Print and shaded views of the part. All mm, measured from the part's lowest x, y and z. Coordinates: 2 decimals unless noted, no trailing zeros. Loops run counter-clockwise (first coordinate to the right, second up) from the corner with the lowest first, then second, coordinate; pieces in that order, holes last.
1) Two-plate mould, pull along Z, no slides. Class the marked faces 1, 2, 3 and 4: +Z half, -Z half, draft (parallel to the pull), parting line (faces both ways), or undercut.
2) Saw through at B-B, the plane y = 1.5. Write the cut outline in (x, z) (1 decimal), and give its area (3 significant figures).
3) Wall check: line 1 along Z through (x, y) = (5.75, 4.25) (1 decimal); line 2 along Y through (x, z) = (11.25, 2.5) (1 decimal); line 3 along X through (y, z) = (3, 4.5). Give the ranges that are in metal, low to high.
4) Pin check, flat tips, straight feed: pin 1 Ø2.5 at (x, z) = (21, 20.5) entering from -Y (3 decimals); pin 2 Ø4 at (x, z) = (7, 3.5) entering from +Y (3 decimals). Stop position of each tip, or through.
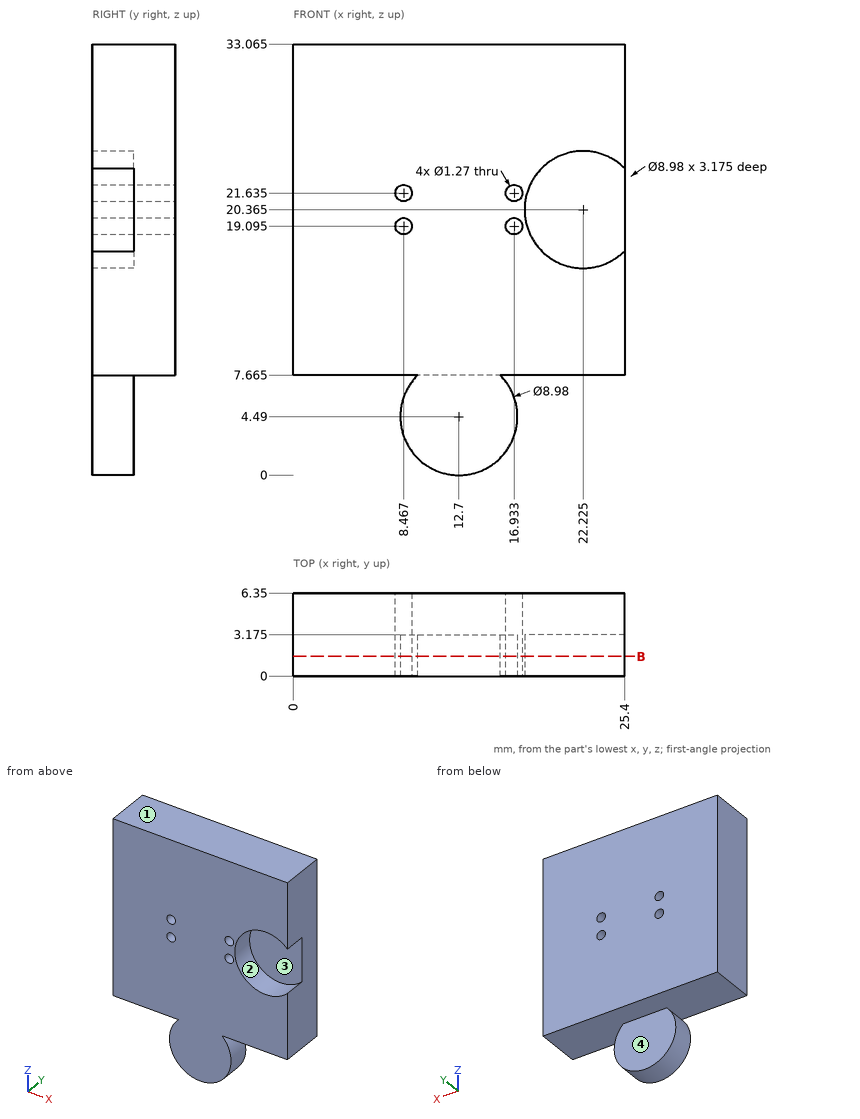
Data:
1. face 1: +Z half
1. face 2: undercut
1. face 3: undercut
1. face 4: draft
2. outline: (0, 7.7) - (9.5, 7.7) arc R4.5 ccw (long way) to (15.9, 7.7) - (25.4, 7.7) - (25.4, 17.2) arc R4.5 cw (long way) to (25.4, 23.5) - (25.4, 33.1) - (0, 33.1) - close; hole circle Ø1.3 at (8.5, 19.1); hole circle Ø1.3 at (8.5, 21.6); hole circle Ø1.3 at (16.9, 19.1); hole circle Ø1.3 at (16.9, 21.6)
2. area: 640 mm2
3. line 1: z = 7.7 to 33.1
3. line 2: y = 0 to 3.2
3. line 3: x = 8.21 to 17.19
4. pin 1: stops at y = 3.175
4. pin 2: stops at y = 3.175
